```python
from build123d import *

# Parameters (mm, degrees)
SKETCH1_R           = 14.65
SKETCH1_R_2         = 5
SKETCH1_R_3         = 3.95
BOSS_EXTRUDE1_DEPTH = 240
SKETCH1_3_R         = 5
BOSS_EXTRUDE2_DEPTH = 14.5
BOSS_EXTRUDE3_START = -14.5
SKETCH1_4_R         = 3.95
BOSS_EXTRUDE3_DEPTH = 12.3
BOSS_EXTRUDE4_START = 261.7
SKETCH1_5_R         = 5
SKETCH1_5_R_2       = 3.95
BOSS_EXTRUDE4_DEPTH = 21.7
BOSS_EXTRUDE5_START = 283.3
SKETCH1_6_R         = 3.95
BOSS_EXTRUDE5_DEPTH = 21.6


with BuildPart() as part:
    # Sketch1 → Boss-Extrude1 (new body)
    # profile 1 of 3: a face of its own
    with BuildSketch(Plane.XY):
        Circle(SKETCH1_R)
        Circle(SKETCH1_R_2, mode=Mode.SUBTRACT)
    # profile 2 of 3: a face of its own
    with BuildSketch(Plane.XY):
        Circle(SKETCH1_R_2)
        Circle(SKETCH1_R_3, mode=Mode.SUBTRACT)
    # profile 3 of 3: a face of its own
    with BuildSketch(Plane.XY):
        Circle(SKETCH1_R_3)
    extrude(amount=BOSS_EXTRUDE1_DEPTH)

    # Sketch1<3> → Boss-Extrude2 (add)
    with BuildSketch(Plane.XY):
        Circle(SKETCH1_3_R)
    extrude(amount=-BOSS_EXTRUDE2_DEPTH)

    # Sketch1<4> → Boss-Extrude3 (add)
    with BuildSketch(Plane.XY.offset(BOSS_EXTRUDE3_START)):
        Circle(SKETCH1_4_R)
    extrude(amount=-BOSS_EXTRUDE3_DEPTH)

    # Sketch1<5> → Boss-Extrude4 (add)
    # profile 1 of 2: a face of its own
    with BuildSketch(Plane.XY.offset(BOSS_EXTRUDE4_START)):
        Circle(SKETCH1_5_R)
        Circle(SKETCH1_5_R_2, mode=Mode.SUBTRACT)
    # profile 2 of 2: a face of its own
    with BuildSketch(Plane.XY.offset(BOSS_EXTRUDE4_START)):
        Circle(SKETCH1_5_R_2)
    extrude(amount=-BOSS_EXTRUDE4_DEPTH)

    # Sketch1<6> → Boss-Extrude5 (add)
    with BuildSketch(Plane.XY.offset(BOSS_EXTRUDE5_START)):
        Circle(SKETCH1_6_R)
    extrude(amount=-BOSS_EXTRUDE5_DEPTH)


solid = part.part
```
Check sheet for the modelled part. Datum: model origin and axes. Units: mm. A direction names the side the tool comes from. Round coordinates to 2 decimals unless told otherwise and drop trailing zeros. Write each loop counter-clockwise with the first axis right and the second up, starting at its lowest first coordinate (ties: lowest second). Pieces come first, ordered by that corner, then holes. Notation, with made-up numbers: (39, 43.5) -> (74, 43.5) arc R28 cw to (74, 70.5) -> close; hole circle Ø3 at (-29, 12.25). An arc over 180 degrees is marked (long way). One line per question, with ' | ' between items. Start each with the question number.
1. Sectioned sample at C-C, the plane z = -4. Record the cut outline in (x, y).
2. Depth check by flat-ended pin: pin 1 (6 mm diameter, centred on x = -5, y = -6.5, fed in from +Z); pin 2 (6 mm diameter, centred on y = 4, z = 141.5, fed in from +X); pin 3 (2 mm diameter, centred on y = 4.5, z = 225, fed in from +X); pin 4 (10 mm diameter, centred on y = -1.5, z = 74.5, fed in from -X). Enter the tip coordinate at first touch or a pass-through.
3. Scan lines: line 1 along Z through (x, y) = (-7.5, -5.5); line 2 along Y through (x, z) = (-0.25, 145.5); line 3 along Y through (x, z) = (-12, 231.5). Record each from-to range of solid material in increasing order. Write a range as from..to.
4. Set-up check for faces 1 (the face through (6, 0, 240)), 2 (the face through (4, 2, -14.5)), 3 (the face through (0, 0, -26.8)): record each of +Z, -Z, +X, -X, +Y, -Y from which the full face is reachable in a straight line by a thin tool's end or side.
5. Sectioned sample at D-D, the plane z = 37. Record the cut outline in (x, y).
6. Sectioned sample at A-A, the plane y = 0. Record the cut outline in (x, z), then the cut area to 3 significant figures.
Taken from the geometry:
1) outline: circle Ø10 at (0, 0)
2) pin 1: stops at z = 240 | pin 2: stops at x = 14.62 | pin 3: stops at x = 14.23 | pin 4: stops at x = -14.65
3) line 1: z = 0..240 | line 2: y = -14.65..14.65 | line 3: y = -8.4..8.4
4) face 1: +Z | face 2: -Z | face 3: -Z, +X, -X, +Y, -Y
5) outline: circle Ø29.3 at (0, 0)
6) outline: (-14.65, 0) -> (-5, 0) -> (-5, -14.5) -> (-3.95, -14.5) -> (-3.95, -26.8) -> (3.95, -26.8) -> (3.95, -14.5) -> (5, -14.5) -> (5, 0) -> (14.65, 0) -> (14.65, 240) -> (5, 240) -> (5, 261.7) -> (3.95, 261.7) -> (3.95, 283.3) -> (-3.95, 283.3) -> (-3.95, 261.7) -> (-5, 261.7) -> (-5, 240) -> (-14.65, 240) -> close | area: 7,660 mm^2
